Work out the finished part from the listing and answer in its coordinate system (mm). A direction names the side the tool comes from. Give positions to 0.01 mm unless a question says otherwise; leave off trailing zeros. Loops run counter-clockwise (first coordinate to the right, second up) from the corner with the lowest first, then second, coordinate; pieces in that order, holes last. Notation, with made-up numbers: M 33,27.5 L 38,27.5 A17 ccw 38,33.5 Z; hole C 53,-14.5 d7. An arc over 180 degrees is marked long. Use a Markdown table: item, result.
```python
from build123d import *

# Parameters (mm, degrees)
F0_R      = 15
F1_DEPTH  = 40
F2_R      = 25.4542264432
F2_R_2    = 13.5
F3_DEPTH  = 34
F4_R      = 18.7341307963
F4_R_2    = 13.5
F5_DEPTH  = 3
F6_R      = 6
F7_DEPTH  = 40.001
F8_R      = 2.85
F9_DEPTH  = 40.001
F10_R     = 2.85
F11_DEPTH = 40.001
F12_R     = 2.15
F13_DEPTH = 20
F14_R     = 3
F15_DEPTH = 18
F17_R     = 2
F18_DEPTH = 11.5


with BuildPart() as f1:
    # F0 (on Front) → F1 (new body)
    with BuildSketch(Plane.XZ):
        Circle(F0_R)
    extrude(amount=-F1_DEPTH)

    # F2 (on face) → F3 (cut)
    with BuildSketch(Plane.XZ):
        Circle(F2_R)
        Circle(F2_R_2, mode=Mode.SUBTRACT)
    extrude(amount=-F3_DEPTH, mode=Mode.SUBTRACT)

    # F4 (on face) → F5 (cut)
    with BuildSketch(Plane(origin=(0, 40, 0), x_dir=(-1, 0, 0), z_dir=(0, 1, 0))):
        Circle(F4_R)
        Circle(F4_R_2, mode=Mode.SUBTRACT)
    extrude(amount=-F5_DEPTH, mode=Mode.SUBTRACT)

    # F6 (on face) → F7 (cut, through all)
    with BuildSketch(Plane.XZ):
        with Locations((5, 0)):
            Circle(F6_R)
    extrude(amount=-F7_DEPTH, mode=Mode.SUBTRACT)

    # F8 (on face) → F9 (cut, through all)
    with BuildSketch(Plane.XZ):
        with Locations((-4.87, -6.95)):
            Circle(F8_R)
    extrude(amount=-F9_DEPTH, mode=Mode.SUBTRACT)

    # F10 (on face) → F11 (cut, through all)
    with BuildSketch(Plane.XZ):
        with Locations((-8.5, 0)):
            Circle(F10_R)
    extrude(amount=-F11_DEPTH, mode=Mode.SUBTRACT)

    # F12 (on face) → F13 (cut)
    with BuildSketch(Plane.XZ):
        with Locations((-7.6642647059, 6.3451986981)):
            Circle(F12_R)
    extrude(amount=-F13_DEPTH, mode=Mode.SUBTRACT)

    # F14 (on face) → F15 (cut)
    with BuildSketch(Plane(origin=(0, 40, 0), x_dir=(-1, 0, 0), z_dir=(0, 1, 0))):
        with Locations((4.62, 7.15)):
            Circle(F14_R)
    extrude(amount=-F15_DEPTH, mode=Mode.SUBTRACT)

    # F17 (on offset) → F18 (cut)
    with BuildSketch(Plane.XY.offset(13.75)):
        with Locations((0, 5)):
            Circle(F17_R)
    extrude(amount=-F18_DEPTH, mode=Mode.SUBTRACT)

    # F20 (on offset) → F21 (revolve, cut)
    with BuildSketch(Plane.XZ.offset(-5)):
        Polygon((5.2748702346, -12.4268155216), (2.9304834637, -6.9037864009), (1.0894737568, -7.6852486579), (3.4338605277, -13.2082777786), align=None)
    revolve(axis=Axis((2.6374351173, 5, -6.2134077608), (0.3907311285, 0, -0.9205048535)), mode=Mode.SUBTRACT)


solid = f1.part
```
(1) Which of the six approach directions +Z, -Z, +X, -X, +Y, -Y give full straight-line access (tool end or side, diameter ignored) to faces 5 (the cylindrical face through (-10.713, 16.762, -8.215)), 6 (the cylindrical face through (2.93, 38.52, -13.18)), 7 (the flat face through (-3, 0, 0)), 8 (the cylindrical face through (-2, 5, 8)), 9 (the flat face through (-3, 40, 0))?
Entries:
| item | result |
|---|---|
| face 5 | -Y |
| face 6 | +Y |
| face 7 | +Z, -Z, +X, -X, -Y |
| face 8 | +Z |
| face 9 | +Z, -Z, +X, -X, +Y |
(2) The mould has two halves that part along Y. Classify faces 1 (the flat face through (-5, 22, 7)), 2 (the flat face through (-1, 5, 2.25)), 3 (the flat face through (-11.18, 34, 7.85)), 4 (the flat face through (2.905, 5.028, -6.915)): released by +Y, released by -Y, zero draft, split by the parting line, or undercut.
Entries:
| item | result |
|---|---|
| face 1 | released by +Y |
| face 2 | undercut |
| face 3 | released by -Y |
| face 4 | undercut |
(3) A cutting plane is placed at D-D (y = 5). Write down the section's boundary in (x, z).
Entries:
| item | result |
|---|---|
| outline | M -2,2.25 L -2,13.35 A13.5 ccw long 3.38,-13.07 L 1.09,-7.69 L 4.77,-6.12 L 7.06,-11.51 A13.5 ccw 2,13.35 L 2,5.2 A6 cw long -0.56,2.25 Z; hole C -8.5,0 d5.7; hole C -7.66,6.35 d4.3; hole C -4.87,-6.95 d5.7 |
(4) A cutting plane is placed at C-C (x = -9). Write down the section's boundary in (y, z).
Entries:
| item | result |
|---|---|
| outline | M 0,-10.06 L 34,-10.06 L 34,-12 L 37,-12 L 37,-10.06 L 40,-10.06 L 40,-2.81 L 0,-2.81 Z; M 0,2.81 L 40,2.81 L 40,10.06 L 37,10.06 L 37,12 L 34,12 L 34,10.06 L 0,10.06 L 0,8.03 L 20,8.03 L 20,4.66 L 0,4.66 Z |
(5) A cutting plane is placed at B-B (y = 24). Write down the section's boundary in (x, z).
Entries:
| item | result |
|---|---|
| outline | C 0,0 d27; hole C -8.5,0 d5.7; hole C -4.87,-6.95 d5.7; hole C -4.62,7.15 d6; hole C 5,0 d12 |
(6) Consider probe 1 along Z at (x, y) = (-4.62, 33.5); probe 2 along Y at (x, z) = (-1.5, 11.25); probe 3 along Y at (x, z) = (-3.25, 5). Determine where each line is inside the solid, lowest interval first. Write a range as [from, to].
Entries:
| item | result |
|---|---|
| probe 1 | z = [-12.68, -9.79], [-4.11, 4.15], [10.15, 12.68] |
| probe 2 | y = [0, 3.68], [6.32, 40] |
| probe 3 | y = [0, 22] |
(7) A cutting plane is placed at A-A (z = 0). Write down the section's boundary in (x, y).
Entries:
| item | result |
|---|---|
| outline | M -15,34 L -13.5,34 L -13.5,0 L -11.35,0 L -11.35,40 L -13.5,40 L -13.5,37 L -15,37 Z; M -5.65,0 L -1,0 L -1,40 L -5.65,40 Z; M 11,0 L 13.5,0 L 13.5,34 L 15,34 L 15,37 L 13.5,37 L 13.5,40 L 11,40 Z |
(8) Given P1, Ø3, axis at x = 0, y = 5, coming from the -Z side; P2, Ø6, axis at y = 16, z = -4, coming from the -X side; P3, Ø1.5, axis at x = 5, y = 11, coming from the -Z side, each flat-ended and moving along its own axis, determine where each tip first touches the part or whether it passes through.
Entries:
| item | result |
|---|---|
| P1 | stops at z = -13.5 |
| P2 | stops at x = -13.46 |
| P3 | stops at z = -12.81 |
